from build123d import *

# Parameters (mm, degrees)
BOSS_EXTRUDE1_START = -2
SKETCH1_R           = 30
SKETCH1_R_2         = 27.5
BOSS_EXTRUDE1_DEPTH = 37.9
SKETCH2_R           = 28.8
CUT_EXTRUDE1_DEPTH  = 2
SKETCH3_R           = 28.8
CUT_EXTRUDE2_DEPTH  = 2
SKETCH5_R           = 26
CUT_EXTRUDE3_DEPTH  = 38.9


with BuildPart() as part:
    # Sketch1 → Boss-Extrude1 (new body)
    with BuildSketch(Plane.XY.offset(BOSS_EXTRUDE1_START)):
        with Locations((0, -108.5)):
            Circle(SKETCH1_R)
        with Locations((0, -108.5)):
            Circle(SKETCH1_R_2, mode=Mode.SUBTRACT)
    extrude(amount=-BOSS_EXTRUDE1_DEPTH)

    # Sketch2 → Cut-Extrude1 (cut)
    with BuildSketch(Plane.XY.offset(-2)):
        with Locations((0, -108.5)):
            Circle(SKETCH2_R)
    extrude(amount=-CUT_EXTRUDE1_DEPTH, mode=Mode.SUBTRACT)

    # Sketch3 → Cut-Extrude2 (cut)
    with BuildSketch(Plane(origin=(0, 0, -39.9), x_dir=(-1, 0, 0), z_dir=(0, 0, -1))):
        with Locations((0, -108.5)):
            Circle(SKETCH3_R)
    extrude(amount=-CUT_EXTRUDE2_DEPTH, mode=Mode.SUBTRACT)

    # Sketch4 → Revolve1 (revolve)
    with BuildSketch(Plane(origin=(0, 0, 0), x_dir=(0, 0, -1), z_dir=(1, 0, 0))):
        Polygon((20.95, -79.75), (20.95, -83.75), (18.45, -83.75), align=None)
    revolve(axis=Axis((0, -79.75, -20.95), (0, -1, 0)))

    # Sketch5 → Cut-Extrude3 (cut, through all)
    with BuildSketch(Plane.XY.offset(-2)):
        with Locations((0, -108.5)):
            Circle(SKETCH5_R)
    extrude(amount=-CUT_EXTRUDE3_DEPTH, mode=Mode.SUBTRACT)


solid = part.part
The listing builds one solid part. Answer for the finished solid, in the listing's coordinates (mm). A direction names the side the tool comes from. Give positions to 0.01 mm unless a question says otherwise; leave off trailing zeros. Loops run counter-clockwise (first coordinate to the right, second up) from the corner with the lowest first, then second, coordinate; pieces in that order, holes last. Notation, with made-up numbers: (9, 42) - (50, 42) arc R20 cw to (50, 77) - close; hole circle Ø1 at (47, 73.25). An arc over 180 degrees is marked (long way). Answer as a JSON object with one key per item and string values.
1. A cutting plane is placed at D-D (z = -20.95). Write down the section's boundary in (x, y).
Determined:
{"outline": "circle Ø60 at (0, -108.5); hole (-1.76, -82.56) - (-0.79, -81.01) arc R27.5 ccw (long way) to (0.79, -81.01) - (1.76, -82.56) arc R26 ccw to start"}
2. Find the intervals of material crossed by L1, parallel to X at y = -108, z = -38; L2, parallel to Y at x = 0, z = -39.05; L3, parallel to Y at x = 0.5, z = -10, in increasing order. Write a range as [from, to].
Determined:
{"L1": "[-30, -28.8], [28.8, 30]", "L2": "[-138.5, -137.3], [-79.7, -78.5]", "L3": "[-138.5, -136], [-81, -78.5]"}
3. A cutting plane is placed at C-C (z = -16.5). Write down the section's boundary in (x, y), then the cut area to 3 significant figures.
Determined:
{"outline": "circle Ø60 at (0, -108.5); hole circle Ø55 at (0, -108.5)", "area": "452 mm²"}
4. A cutting plane is placed at B-B (x = -15). Write down the section's boundary in (y, z).
Determined:
{"outline": "(-134.48, -39.9) - (-133.09, -39.9) - (-133.09, -37.9) - (-131.55, -37.9) - (-131.55, -4) - (-133.09, -4) - (-133.09, -2) - (-134.48, -2) - close; (-85.45, -37.9) - (-83.91, -37.9) - (-83.91, -39.9) - (-82.52, -39.9) - (-82.52, -2) - (-83.91, -2) - (-83.91, -4) - (-85.45, -4) - close"}
5. For a pull along X with two mould halves and no side action, classify faces 1 (the cylindrical face through (-6.503, -137.787, -20.685)), 2 (the flat face through (-11.3, -81.7, -2)), 3 (the flat face through (-11, -134, -37.9)) as pulls with the +X half, pulls with the -X half, needs draft (parallel to the pull), parting line crosses it, or undercut.
Determined:
{"face 1": "parting line crosses it", "face 2": "needs draft", "face 3": "undercut"}
6. For faces 4 (the conical face through (-0.633, -81.249, -21.641)), 5 (the cylindrical face through (0, -82.5, -20.9)), 6 (the flat face through (11, -134, -4)), 7 (the cylindrical face through (-13.29, -134.05, -38.91)), determine the directions among +Z, -Z, +X, -X, +Y, -Y from which every point of the face is accessible in a straight line to the end or side of a thin tool.
Determined:
{"face 4": "none", "face 5": "+Z, -Z", "face 6": "+Z", "face 7": "-Z"}
7. A cutting plane is placed at A-A (y = -108.5). Write down the section's boundary in (x, z).
Determined:
{"outline": "(-30, -39.9) - (-28.8, -39.9) - (-28.8, -37.9) - (-27.5, -37.9) - (-27.5, -4) - (-28.8, -4) - (-28.8, -2) - (-30, -2) - close; (27.5, -37.9) - (28.8, -37.9) - (28.8, -39.9) - (30, -39.9) - (30, -2) - (28.8, -2) - (28.8, -4) - (27.5, -4) - close"}
8. Flat-ended cylindrical pins translate along their axes: pin 1 Ø1.5 at (x, z) = (15, -30.5) entering from -Y; pin 2 Ø10 at (y, z) = (-91, -24.5) entering from +X; pin 3 Ø12 at (y, z) = (-91, -33.5) entering from +X. Find the tip coordinate at first contact, or state that the pin passes through.
Determined:
{"pin 1": "y = -134.9", "pin 2": "x = 27.27", "pin 3": "x = 27.71"}
